from build123d import *

# Parameters (mm, degrees)
F0_W     = 9.8080858588
F0_H     = 15.6037732959
F0_W_2   = 28.9784371853
F0_H_2   = 41.4614528418
F0_W_3   = 15.1579454541
F0_H_3   = 8.9164413512
F1_DEPTH = 25.4


with BuildPart() as f1:
    # F0 (on Front) → F1 (new body)
    with BuildSketch(Plane.XZ):
        Polygon((-47.0342300832, 34.1053940356), (-57.7339567244, 34.1053940356), (-57.7339567244, -31.8762771785), (29.6471677721, -31.8762771785), (29.6471677721, 34.1053940356), (-37.2261442244, 34.1053940356), align=None)
        Polygon((-57.7339567244, -31.8762771785), (-57.7339567244, 34.1053940356), (-85.820749402, -31.8762771785), align=None)
        with Locations((-42.1301871538, 41.9072806835)):
            Rectangle(F0_W, F0_H)
        with BuildLine():
            Line((29.6471677721, -31.8762771785), (-57.7339567244, -31.8762771785))
            Line((-57.7339567244, -31.8762771785), (-85.820749402, -31.8762771785))
            Line((-85.820749402, -31.8762771785), (-85.820749402, -41.6843593121))
            Line((-85.820749402, -41.6843593121), (-65.7587572932, -41.6843593121))
            ThreePointArc((-65.7587572932, -41.6843593121), (-61.7463588715, -41.3036522536), (-57.7339604497, -41.6843593121))
            Line((-57.7339604497, -41.6843593121), (75.566843152, -41.6843593121))
            Line((75.566843152, -41.6843593121), (75.566843152, -31.8762771785))
            Line((75.566843152, -31.8762771785), (29.6471677721, -31.8762771785))
        make_face()
        Polygon((-85.820749402, -41.6843593121), (-85.820749402, -31.8762771785), (-111.2326085567, -49.9320700765), (-85.820749402, -49.9320700765), align=None)
        Polygon((-50.6008081138, 49.7091673315), (-47.0342300832, 49.7091673315), (-37.2261442244, 49.7091673315), (-34.1053903103, 49.7091673315), (-34.1053903103, 55.059030652), (-50.6008081138, 55.059030652), align=None)
        Polygon((29.6471677721, 34.1053940356), (29.6471677721, -31.8762771785), (75.566843152, -31.8762771785), (76.0126635432, -31.8762771785), (76.0126635432, -20.2849023044), (76.0126635432, -11.3684609532), (76.0126635432, 76.0126635432), (29.6471677721, 76.0126635432), align=None)
        with Locations((53.0528277159, 39.6781675518)):
            Rectangle(F0_W_2, F0_H_2, mode=Mode.SUBTRACT)
        with BuildLine():
            Line((-65.7587572932, -41.6843593121), (-85.820749402, -41.6843593121))
            Line((-85.820749402, -41.6843593121), (-85.820749402, -49.9320700765))
            Line((-85.820749402, -49.9320700765), (-85.820749402, -58.1797808409))
            Line((-85.820749402, -58.1797808409), (-82.6096979015, -58.1797808409))
            ThreePointArc((-82.6096979015, -58.1797808409), (-76.6703433025, -47.3923721355), (-65.7587572932, -41.6843593121))
        make_face()
        Polygon((-85.820749402, -49.9320700765), (-111.2326085567, -49.9320700765), (-111.2326085567, -67.0962259173), (-85.820749402, -67.0962259173), (-85.820749402, -58.1797808409), align=None)
        with BuildLine():
            Line((-57.7339604497, -41.6843593121), (-65.7587572932, -41.6843593121))
            ThreePointArc((-65.7587572932, -41.6843593121), (-76.6703433025, -47.3923721355), (-82.6096979015, -58.1797808409))
            Line((-82.6096979015, -58.1797808409), (-40.8830198414, -58.1797808409))
            ThreePointArc((-40.8830198414, -58.1797808409), (-46.8223744405, -47.3923721355), (-57.7339604497, -41.6843593121))
        make_face()
        Polygon((14.0433991328, 76.0126635432), (29.6471677721, 76.0126635432), (76.0126635432, 76.0126635432), (91.1706089973, 76.0126635432), (91.1706089973, 86.2665772438), (14.0433991328, 86.2665772438), align=None)
        with BuildLine():
            Line((76.0126635432, -41.6843593121), (75.566843152, -41.6843593121))
            Line((75.566843152, -41.6843593121), (-57.7339604497, -41.6843593121))
            ThreePointArc((-57.7339604497, -41.6843593121), (-46.8223744405, -47.3923721355), (-40.8830198414, -58.1797808409))
            Line((-40.8830198414, -58.1797808409), (-38.0569003573, -58.1797808409))
            ThreePointArc((-38.0569003573, -58.1797808409), (-18.5016151518, -42.2295010715), (1.0536700538, -58.1797808409))
            Line((1.0536700538, -58.1797808409), (3.4778552674, -58.1797808409))
            ThreePointArc((3.4778552674, -58.1797808409), (23.4056599438, -42.2175962213), (43.3334646202, -58.1797808409))
            Line((43.3334646202, -58.1797808409), (44.805124402, -58.1797808409))
            ThreePointArc((44.805124402, -58.1797808409), (57.210420743, -43.8584153697), (76.0126635432, -46.19690889))
            Line((76.0126635432, -46.19690889), (76.0126635432, -41.6843593121))
        make_face()
        with BuildLine():
            Line((-40.8830198414, -58.1797808409), (-82.6096979015, -58.1797808409))
            ThreePointArc((-82.6096979015, -58.1797808409), (-63.9878782959, -83.8542812252), (-40.4120040206, -62.6380071044))
            ThreePointArc((-40.4120040206, -62.6380071044), (-40.5300847506, -60.39648768), (-40.8830198414, -58.1797808409))
        make_face()
        with Locations((83.5916362703, -15.8266816288)):
            Rectangle(F0_W_3, F0_H_3)
        Polygon((91.1706089973, -11.3684609532), (91.1706089973, -20.2849023044), (91.1706089973, -24.74312298), (98.3037799597, -24.74312298), (98.3037799597, -6.4644180238), (91.1706089973, -6.4644180238), align=None)
        with BuildLine():
            ThreePointArc((84.5376919751, -62.6380071044), (82.2797104052, -53.3780689261), (76.0126635432, -46.19690889))
            Line((76.0126635432, -46.19690889), (76.0126635432, -58.1797808409))
            Line((76.0126635432, -58.1797808409), (44.805124402, -58.1797808409))
            ThreePointArc((44.805124402, -58.1797808409), (62.1781869933, -82.6289594789), (84.5376919751, -62.6380071044))
        make_face()
        with BuildLine():
            Line((76.0126635432, -58.1797808409), (76.0126635432, -46.19690889))
            ThreePointArc((76.0126635432, -46.19690889), (57.210420743, -43.8584153697), (44.805124402, -58.1797808409))
            Line((44.805124402, -58.1797808409), (76.0126635432, -58.1797808409))
        make_face()
        with BuildLine():
            ThreePointArc((1.0536700538, -58.1797808409), (-18.5016151518, -42.2295010715), (-38.0569003573, -58.1797808409))
            Line((-38.0569003573, -58.1797808409), (1.0536700538, -58.1797808409))
        make_face()
        with BuildLine():
            Line((1.0536700538, -58.1797808409), (-38.0569003573, -58.1797808409))
            ThreePointArc((-38.0569003573, -58.1797808409), (-20.5181288599, -82.0527480619), (1.4610630394, -62.1921792626))
            ThreePointArc((1.4610630394, -62.1921792626), (1.3589536475, -60.1756655545), (1.0536700538, -58.1797808409))
        make_face()
        with BuildLine():
            ThreePointArc((43.826070827, -62.6380071044), (43.7025456671, -60.3953277754), (43.3334646202, -58.1797808409))
            Line((43.3334646202, -58.1797808409), (3.4778552674, -58.1797808409))
            ThreePointArc((3.4778552674, -58.1797808409), (21.1629806148, -82.9348928277), (43.826070827, -62.6380071044))
        make_face()
        with BuildLine():
            Line((3.4778552674, -58.1797808409), (43.3334646202, -58.1797808409))
            ThreePointArc((43.3334646202, -58.1797808409), (23.4056599438, -42.2175962213), (3.4778552674, -58.1797808409))
        make_face()
    extrude(amount=F1_DEPTH)


solid = f1.part
Input: part model. Units: mm. Frame: model coordinates. A direction names the side the tool comes from. Coordinates: 2 decimals unless noted, no trailing zeros. Loops run counter-clockwise (first coordinate to the right, second up) from the corner with the lowest first, then second, coordinate; pieces in that order, holes last.
Q1. Contact query for flat-ended pins moving along their axis: pin 1 (12 mm diameter, centred on x = -58, z = -52, fed in from +Y); pin 2 (1.1 mm diameter, centred on x = -49.5, y = -7.5, fed in from -Z); pin 3 (10 mm diameter, centred on x = -59, y = -20, fed in from +Z); pin 4 (8 mm diameter, centred on x = -45, y = -7, fed in from +Z). Output: stop coordinate, or through.
Q2. Cut plane C-C (x = 52). Output: boundary loops of the cut face in (y, z), then the cut area to 3 significant figures.
Q3. Material intervals for line 1 (X direction, y = -11.25, z = 37); line 2 (X direction, y = -17.75, z = 33); line 3 (Z direction, x = 23, y = -21), sorted ascending.
Q4. Cut plane D-D (z = 1.5). Output: boundary loops of the cut face in (x, y), then the cut area to 3 significant figures.
Q5. Cut plane A-A (x = 22). Output: boundary loops of the cut face in (y, z), then the cut area to 3 significant figures.
Q6. Draft query along Z for faces 1 (the face through (83, -13, -20.285)), 2 (the face through (-42, -13, 55.059)), 3 (the face through (-99, -13, -67.096)). Return one class per face: +Z half, -Z half, draft (parallel to the pull), parting line (faces both ways), or undercut.
Q7. Cut plane B-B (y = -19.5). Give the number of separate pieces and of enclosed holes in the cut face, then the cut area to 3 significant figures.
Q8. Set-up query: faces 4 (the face through (91.171, -13, 81)), 5 (the face through (75.567, -13, -37)), 6 (the face through (53, -13, 18.947)), 7 (the face through (-47.034, -13, 42)), 8 (the face through (91.171, -13, -22)). Return all of +Z, -Z, +X, -X, +Y, -Y with unobstructed straight access to the full face (end or side cutting, diameter ignored); none if empty.
Working result:
1. pin 1: stops at y = 0
1. pin 2: stops at z = -80.48
1. pin 3: stops at z = 34.11
1. pin 4: stops at z = 55.06
2. outline: (-25.4, -78.46) - (0, -78.46) - (0, 18.95) - (-25.4, 18.95) - close; (-25.4, 60.41) - (0, 60.41) - (0, 86.27) - (-25.4, 86.27) - close
2. area: 3,130 mm2
3. line 1: x = -47.03 to -37.23, 29.65 to 38.56, 67.54 to 76.01
3. line 2: x = -58.2 to 38.56, 67.54 to 76.01
3. line 3: z = -83.05 to 34.11, 76.01 to 86.27
4. outline: (-71.61, -25.4) - (76.01, -25.4) - (76.01, 0) - (-71.61, 0) - close
4. area: 3,750 mm2
5. outline: (-25.4, -83.01) - (0, -83.01) - (0, 34.11) - (-25.4, 34.11) - close; (-25.4, 76.01) - (0, 76.01) - (0, 86.27) - (-25.4, 86.27) - close
5. area: 3,240 mm2
6. face 1: undercut
6. face 2: +Z half
6. face 3: -Z half
7. separate pieces: 1
7. enclosed holes: 2
7. area: 20,100 mm2
8. face 4: +Z, +X, +Y, -Y
8. face 5: +X, +Y, -Y
8. face 6: +Y, -Y
8. face 7: -X, +Y, -Y
8. face 8: -Z, +Y, -Y
